```python
from build123d import *

# Parameters (mm, degrees)
F0_W     = 28.184153
F0_H     = 84.810838
F1_DEPTH = 76.2
F2_R     = 7.62
F3_R     = 7.62


with BuildPart() as f1:
    # F0 (on Top) → F1 (new body)
    with BuildSketch(Plane.XY):
        with Locations((-52.143465, -1.344271)):
            Rectangle(F0_W, F0_H)
    extrude(amount=F1_DEPTH)

    # F2
    f2_edges = [f1.edges().sort_by_distance(p)[0] for p in [
        (-66.235542, 41.061148, 38.1),
        (-66.235542, -43.74969, 38.1),
        (-38.051389, -43.74969, 38.1),
        (-38.051389, 41.061148, 38.1),
    ]]
    fillet(f2_edges, radius=F2_R)

    # F3
    f3_edges = [f1.edges().sort_by_distance(p)[0] for p in [
        (-38.051389, -1.344271, 76.2),
        (-66.235542, -1.344271, 76.2),
        (-66.235542, -1.344271, 0),
        (-38.051389, -1.344271, 0),
    ]]
    fillet(f3_edges, radius=F3_R)


solid = f1.part
```
Geometry check sheet. Reference: the model listing, model coordinates, mm. Coordinates: 2 decimals unless noted, no trailing zeros. Order: outer loops, then holes, each group sorted by start corner. A loop starts at its lowest first (then second) coordinate and runs counter-clockwise, first axis right, second up. Notation, with made-up numbers: (53, 83.5) - (89, 83.5) arc R17 cw to (89, 113.5) - close; hole circle Ø1 at (-27.75, 22.5). An arc over 180 degrees is marked (long way). Answer as a JSON object with one key per item and string values. Group by question number.
Item 1: Scan lines: probe 1 along Z at (x, y) = (-59, 3); probe 2 along Z at (x, y) = (-65, -8); probe 3 along Y at (x, z) = (-44, 70). Record each from-to range of solid material in increasing order.
Item 2: Depth check by flat-ended pin: pin 1 Ø1 at (x, z) = (-42.5, 48.5) entering from -Y; pin 2 Ø2 at (x, y) = (-41.5, -33) entering from -Z. Enter the tip coordinate at first touch or a pass-through.
Item 3: Sectioned sample at B-B, the plane z = 9. Record the cut outline in (x, y).
Item 4: Sectioned sample at A-A, the plane y = 26. Record the cut outline in (x, z), and give its area (3 significant figures).
Resolved:
{
 "1": {"probe 1": "0.01 to 76.19", "probe 2": "3.46 to 72.74", "probe 3": "-43.43 to 40.74"},
 "2": {"pin 1": "y = -43.27", "pin 2": "z = 0.69"},
 "3": {"outline": "(-66.24, -36.13) arc R7.62 ccw to (-58.62, -43.75) - (-45.67, -43.75) arc R7.62 ccw to (-38.05, -36.13) - (-38.05, 33.44) arc R7.62 ccw to (-45.67, 41.06) - (-58.62, 41.06) arc R7.62 ccw to (-66.24, 33.44) - close"},
 "4": {"outline": "(-66.24, 7.62) arc R7.62 ccw to (-58.62, 0) - (-45.67, 0) arc R7.62 ccw to (-38.05, 7.62) - (-38.05, 68.58) arc R7.62 ccw to (-45.67, 76.2) - (-58.62, 76.2) arc R7.62 ccw to (-66.24, 68.58) - close", "area": "2,100 mm^2"}
}
